Input: part model. Units: mm. Frame: model coordinates. A direction names the side the tool comes from. Round coordinates to 2 decimals unless told otherwise and drop trailing zeros. Order: outer loops, then holes, each group sorted by start corner. A loop starts at its lowest first (then second) coordinate and runs counter-clockwise, first axis right, second up. Notation, with made-up numbers: (66, 55) -> (103, 55) arc R17 ccw to (103, 87) -> close; hole circle Ø8 at (0, 1.25). An arc over 180 degrees is marked (long way). Use a Markdown table: item, result.
from build123d import *

# Parameters (mm, degrees)
SKETCH8_W          = 20
SKETCH8_H          = 3
SKETCH10_R         = 3
CUT_EXTRUDE1_DEPTH = 50.738672756


with BuildPart() as part:
    # Sweep1: sweep along a path in Sketch7
    with BuildLine(Plane(origin=(0, 0, 0), x_dir=(0, 0, -1), z_dir=(1, 0, 0))) as sweep1_path:
        Line((43.473389189, 0), (23.473389189, 0))
        ThreePointArc((23.473389189, 0), (20.327624841, 1.113592061), (18.583099774, 3.958333333))
        ThreePointArc((18.583099774, 3.958333333), (0, 19), (-18.583099774, 3.958333333))
        ThreePointArc((-18.583099774, 3.958333333), (-20.327624841, 1.113592061), (-23.473389189, 0))
        Line((-23.473389189, 0), (-43.473389189, 0))
    # Sketch8 → Sweep1 (sweep)
    with BuildSketch(Plane.XY.offset(-43.473389189)):
        with Locations((0, 1.5)):
            Rectangle(SKETCH8_W, SKETCH8_H)
    sweep(path=sweep1_path.line)

    # Sketch10 → Cut-Extrude1 (cut, through all)
    with BuildSketch(Plane(origin=(0, 0, 0), x_dir=(-1, 0, 0), z_dir=(0, -1, 0))):
        with Locations(Location((0, 33.473389189, 0), (0, 0, 90))):
            Circle(SKETCH10_R)
        with Locations(Location((0, -33.473389189, 0), (0, 0, 90))):
            Circle(SKETCH10_R)
    extrude(amount=-CUT_EXTRUDE1_DEPTH, mode=Mode.SUBTRACT)


solid = part.part
1) Cut plane D-D on x = -8.25. Return loops of the section in (y, z).
Results found:
| item | result |
|---|---|
| outline | (0, -43.47) -> (3, -43.47) -> (3, -23.47) arc R2 cw to (4.58, -21.52) arc R22 ccw to (4.58, 21.52) arc R2 cw to (3, 23.47) -> (3, 43.47) -> (0, 43.47) -> (0, 23.47) arc R5 ccw to (3.96, 18.58) arc R19 cw to (3.96, -18.58) arc R5 ccw to (0, -23.47) -> close |
2) Cut plane B-B on y = 14.25. Return loops of the section in (x, z).
Results found:
| item | result |
|---|---|
| outline | (-10, -16.76) -> (10, -16.76) -> (10, -12.57) -> (-10, -12.57) -> close; (-10, 12.57) -> (10, 12.57) -> (10, 16.76) -> (-10, 16.76) -> close |
3) Line query: L1, parallel to Y at x = -5.25, z = -29; L2, parallel to Z at x = 5.25, y = 5; L3, parallel to Z at x = 9.25, y = 10.75. Output: solid intervals per line, ascending. Write a range as [from, to].
Results found:
| item | result |
|---|---|
| L1 | y = [0, 3] |
| L2 | z = [-21.42, -18.33], [18.33, 21.42] |
| L3 | z = [-19.19, -15.67], [15.67, 19.19] |
4) Cut plane A-A on x = 0. Return loops of the section in (y, z).
Results found:
| item | result |
|---|---|
| outline | (0, -43.47) -> (3, -43.47) -> (3, -36.47) -> (0, -36.47) -> close; (0, -30.47) -> (3, -30.47) -> (3, -23.47) arc R2 cw to (4.58, -21.52) arc R22 ccw to (4.58, 21.52) arc R2 cw to (3, 23.47) -> (3, 30.47) -> (0, 30.47) -> (0, 23.47) arc R5 ccw to (3.96, 18.58) arc R19 cw to (3.96, -18.58) arc R5 ccw to (0, -23.47) -> close; (0, 36.47) -> (3, 36.47) -> (3, 43.47) -> (0, 43.47) -> close |
5) Pull-direction query (Z, two-part tool) for faces 4 (the flat face through (-2, 0, 36)), 5 (the flat face through (0, 2, -43.473)), 6 (the cylindrical face through (0.14, 1.144, 20.291)); classes: +Z half, -Z half, draft (parallel to the pull), parting line (faces both ways), or undercut.
Results found:
| item | result |
|---|---|
| face 4 | draft |
| face 5 | -Z half |
| face 6 | undercut |
6) Pin query (flat end, axial travel): pin 1 Ø4 at (x, z) = (-2.5, 20) entering from +Y; pin 2 Ø7 at (x, z) = (0, 33.47) entering from +Y; pin 3 Ø1 at (x, y) = (-1.5, 15) entering from +Z; pin 4 Ø3.5 at (x, z) = (0, -33.47) entering from +Y (3 decimals). Return the tip coordinate at first contact, or that it passes through.
Results found:
| item | result |
|---|---|
| pin 1 | stops at y = 12.65 |
| pin 2 | stops at y = 3 |
| pin 3 | stops at z = 16.55 |
| pin 4 | passes through |
7) Set-up query: faces 1 (the flat face through (2, 3, -31)), 2 (the flat face through (2, 3, 36)), 3 (the cylindrical face through (0.14, 1.084, -20.365)). Return all of +Z, -Z, +X, -X, +Y, -Y with unobstructed straight access to the full face (end or side cutting, diameter ignored); none if empty.
Results found:
| item | result |
|---|---|
| face 1 | -Z, +X, -X, +Y |
| face 2 | +Z, +X, -X, +Y |
| face 3 | +X, -X, -Y |
8) Cut plane C-C on z = 34.5. Return loops of the section in (x, y), and give its area (3 significant figures).
Results found:
| item | result |
|---|---|
| outline | (-10, 0) -> (-2.82, 0) -> (-2.82, 3) -> (-10, 3) -> close; (2.82, 0) -> (10, 0) -> (10, 3) -> (2.82, 3) -> close |
| area | 43.1 mm² |
